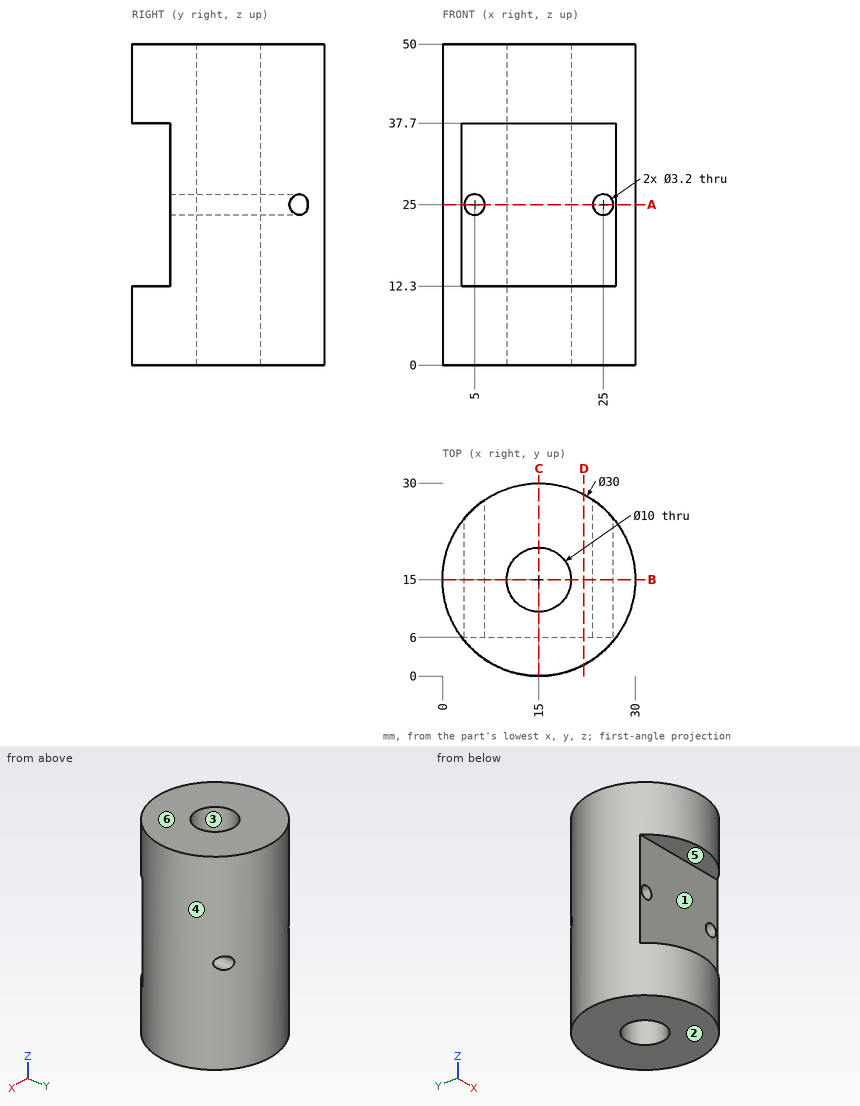
Verification items for this drawing (mm, ordinates from the low corner). A direction names the side the tool comes from. Coordinates: 2 decimals unless noted, no trailing zeros. Write each loop counter-clockwise with the first axis right and the second up, starting at its lowest first coordinate (ties: lowest second). Pieces come first, ordered by that corner, then holes. Notation, with made-up numbers: M 8.25,-6.5 L 12.25,-6.5 A24 cw 12.25,8.5 Z; hole C 13.25,72.5 d11. An arc over 180 degrees is marked long. Answer as CSV lines item,"result".
Q1. Cross-section at C-C (x = 15). Record the boundary of the cut face in (y, z), then the cut area to 3 significant figures.
Check result:
outline,"M 0,0 L 10,0 L 10,50 L 0,50 L 0,37.7 L 6,37.7 L 6,12.3 L 0,12.3 Z; M 20,0 L 30,0 L 30,50 L 20,50 Z"
area,"848 mm^2"
Q2. Set-up check for the marked faces 5 and 6: record each of +Z, -Z, +X, -X, +Y, -Y from which the full face is reachable in a straight line by a thin tool's end or side.
Check result:
face 5,"+X, -X, -Y"
face 6,"+Z, +X, -X, +Y, -Y"
Q3. Material ranges on probe 1 along Y at (x, z) = (15, 24); probe 2 along Z at (x, y) = (5, 26); probe 3 along Z at (x, y) = (17.5, 1), recorded low to high. Write a range as from..to.
Check result:
probe 1,"6..10, 20..30"
probe 2,"0..23.4, 26.6..50"
probe 3,"0..12.3, 37.7..50"
Q4. Go/stop test with flat-tipped pins: pin 1 (5 mm diameter, centred on x = 25, z = 25, fed in from -Y); pin 2 (1.5 mm diameter, centred on x = 18, z = 35, fed in from +Y); pin 3 (5 mm diameter, centred on x = 5, z = 25, fed in from +Y). Record where each tip stops, or that it passes through.
Check result:
pin 1,"y = 6"
pin 2,"y = 29.83"
pin 3,"y = 27.99"
Q5. Cross-section at D-D (x = 22). Record the boundary of the cut face in (y, z), then the cut area to 3 significant figures.
Check result:
outline,"M 1.73,0 L 28.27,0 L 28.27,50 L 1.73,50 L 1.73,37.7 L 6,37.7 L 6,12.3 L 1.73,12.3 Z"
area,"1,220 mm^2"
Q6. Cross-section at B-B (y = 15). Record the boundary of the cut face in (x, z), then the cut area to 3 significant figures.
Check result:
outline,"M 0,0 L 10,0 L 10,50 L 0,50 Z; M 20,0 L 30,0 L 30,50 L 20,50 Z; hole C 5,25 d3.2; hole C 25,25 d3.2"
area,"984 mm^2"
Q7. Mould release check, pull along Y, two halves, no side actions. Record for the marked faces 1, 2, 3 and 4: released by +Y, released by -Y, zero draft, split by the parting line, or undercut.
Check result:
face 1,"released by -Y"
face 2,"zero draft"
face 3,"undercut"
face 4,"split by the parting line"
Q8. Cross-section at A-A (z = 25). Record the boundary of the cut face in (x, y).
Check result:
outline,"M 3,6 L 3.4,6 L 3.4,24.51 A15 ccw Z; M 6.6,6 L 23.4,6 L 23.4,27.43 A15 ccw 6.6,27.43 Z; M 26.6,6 L 27,6 A15 ccw 26.6,24.51 Z; hole C 15,15 d10"
